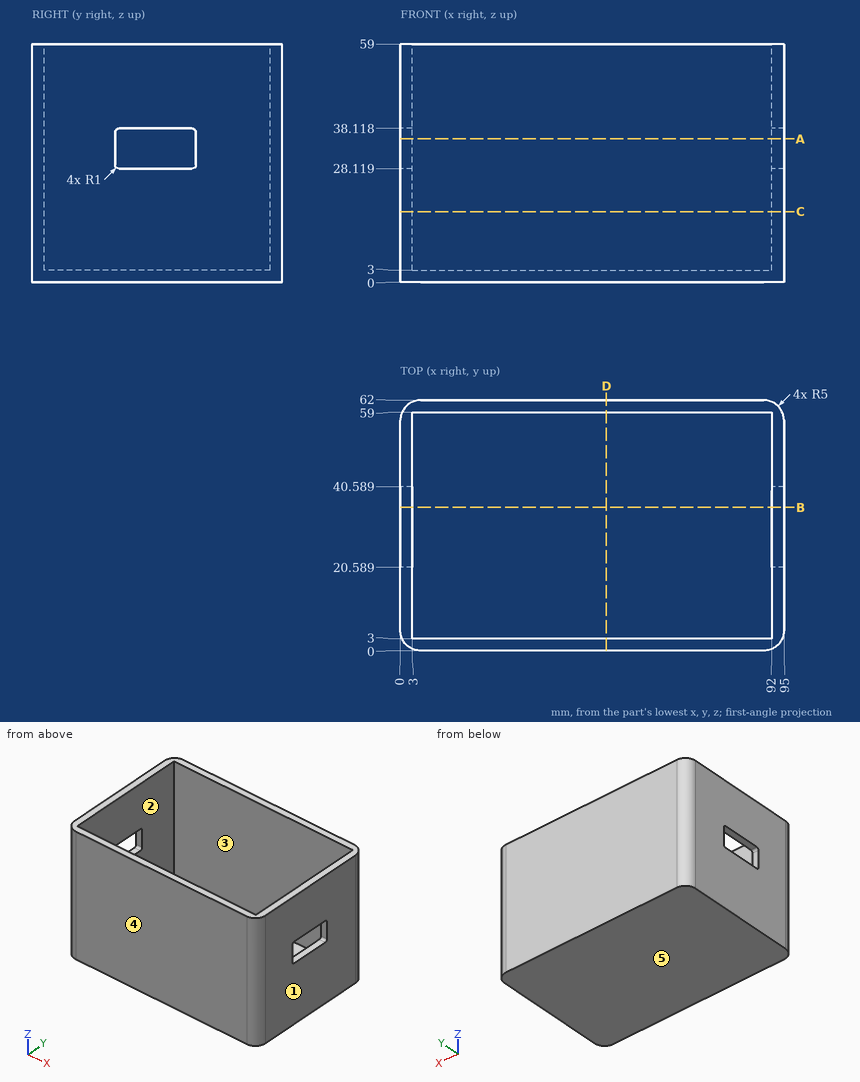
Verification items for this drawing (mm, ordinates from the low corner). A direction names the side the tool comes from. Give positions to 0.01 mm unless a question says otherwise; leave off trailing zeros. Order: outer loops, then holes, each group sorted by start corner. A loop starts at its lowest first (then second) coordinate and runs counter-clockwise, first axis right, second up. Notation, with made-up numbers: M 27,46 L 85,46 A17 ccw 85,68 Z; hole C 76,-18.75 d8. An arc over 180 degrees is marked long. Use a Markdown table: item, result.
Item 1: Draft check along Y on the marked faces 3, 4 and 5. Enter one of: +Y half, -Y half, draft (parallel to the pull), parting line (faces both ways), or undercut.
Answers follow:
| item | result |
|---|---|
| face 3 | undercut |
| face 4 | -Y half |
| face 5 | draft |
Item 2: Material ranges on line 1 along X through (y, z) = (48.5, 53.5); line 2 along Y through (x, z) = (57.5, 38.5); line 3 along Z through (x, y) = (46, 38), recorded low to high.
Answers follow:
| item | result |
|---|---|
| line 1 | x = 0 to 3, 92 to 95 |
| line 2 | y = 0 to 3, 59 to 62 |
| line 3 | z = 0 to 3 |
Item 3: Section check A-A (z = 35.5). Record the cut outline in (x, y).
Answers follow:
| item | result |
|---|---|
| outline | M 0,5 A5 ccw 5,0 L 90,0 A5 ccw 95,5 L 95,20.59 L 92,20.59 L 92,3 L 3,3 L 3,20.59 L 0,20.59 Z; M 0,40.59 L 3,40.59 L 3,59 L 92,59 L 92,40.59 L 95,40.59 L 95,57 A5 ccw 90,62 L 5,62 A5 ccw 0,57 Z |
Item 4: Depth check by flat-ended pin: P1, Ø2.5, axis at x = 94, z = 32.5, coming from the +Y side (1 decimal); P2, Ø3.5, axis at x = 1, z = 31.5, coming from the -Y side (1 decimal); P3, Ø1.5, axis at x = 93.5, z = 34, coming from the -Y side (1 decimal). Enter the tip coordinate at first touch or a pass-through.
Answers follow:
| item | result |
|---|---|
| P1 | stops at y = 61.2 |
| P2 | stops at y = 0.5 |
| P3 | stops at y = 0.8 |
Item 5: Section check C-C (z = 17.5). Record the cut outline in (x, y).
Answers follow:
| item | result |
|---|---|
| outline | M 0,5 A5 ccw 5,0 L 90,0 A5 ccw 95,5 L 95,57 A5 ccw 90,62 L 5,62 A5 ccw 0,57 Z; hole M 3,3 L 92,3 L 92,59 L 3,59 Z |
Item 6: Section check D-D (x = 51). Record the cut outline in (y, z), and give its area (3 significant figures).
Answers follow:
| item | result |
|---|---|
| outline | M 0,0 L 62,0 L 62,59 L 59,59 L 59,3 L 3,3 L 3,59 L 0,59 Z |
| area | 522 mm2 |
Item 7: Section check B-B (y = 35.5). Record the cut outline in (x, z).
Answers follow:
| item | result |
|---|---|
| outline | M 0,0 L 95,0 L 95,28.12 L 92,28.12 L 92,3 L 3,3 L 3,28.12 L 0,28.12 Z; M 0,38.12 L 3,38.12 L 3,59 L 0,59 Z; M 92,38.12 L 95,38.12 L 95,59 L 92,59 Z |
Item 8: Tool access check on the marked faces 1 and 2. Record the directions out of +Z, -Z, +X, -X, +Y, -Y that give a thin tool (end or side, any length) a straight path to the whole face; none if there is none.
Answers follow:
| item | result |
|---|---|
| face 1 | +Z, -Z, +X, +Y, -Y |
| face 2 | +Z |
